Autodesk Inventor part; units mm, degrees
ref_plane "YZ Plane" through (0, 0, 0) normal (1, 0, 0) x (0, 1, 0)
ref_plane "XZ Plane" through (0, 0, 0) normal (0, 1, 0) x (-1, 0, 0)
ref_plane "XY Plane" through (0, 0, 0) normal (0, 0, 1) x (1, 0, 0)
sketch "Sketch1" plane through (0, 0, 0) normal (0, 0, 1) x (1, 0, 0)
  line L0 (0, 0) -> (25.4, 0)
  line L1 (25.4, 0) -> (25.4, 6.35)
  line L2 (25.4, 6.35) -> (0, 6.35)
  line L3 (0, 6.35) -> (0, 0)
  dimension "d0" = 25.4
  dimension "d1" = 6.35
extrude "Extrusion1" add sketch "Sketch1" along normal blind 25.4
sketch "Sketch2" plane through (0, 6.35, 0) normal (0, 1, 0) x (1, 0, 0)
  line L0 (0, 0) -> (25.4, 0)
  line L1 (12.7, 0) -> (12.7, -25.4)
  line L2 (0, -25.4) -> (25.4, -25.4)
  line L3 (0, 0) -> (0, -25.4)
  line L4 (0, -12.7) -> (25.4, -12.7)
  line L5 (25.4, 0) -> (25.4, -25.4)
  line L6 (12.7, -12.7) -> (12.7, -6.35)
  line L7 (12.7, -12.7) -> (12.7, -19.05)
  circle A0 centre (12.7, -6.35) radius 1.5875
  circle A1 centre (12.7, -19.05) radius 1.5875
  dimension "d4" = 6.35
  dimension "d5" = 6.35
  dimension "d6" = 3.175
  dimension "d7" = 3.175
extrude "Extrusion2" cut sketch "Sketch2" against normal blind 25.4 contours A0 L1 | L1 A0 | A1 L1 | L1 A1
sketch "Sketch3" plane through (25.4, 0, 0) normal (1, 0, 0) x (0, 0, -1)
  line L0 (-25.4, 0) -> (-25.4, 6.35)
  line L1 (-25.4, 3.175) -> (0, 3.175)
  line L2 (0, 0) -> (0, 6.35)
  line L3 (-20.6375, 6.35) -> (-20.6375, 0)
  line L4 (-20.6375, 6.35) -> (-20.6375, 3.175)
  line L5 (-4.7625, 6.35) -> (-4.7625, 0)
  line L6 (-4.7625, 6.35) -> (-4.7625, 3.175)
hole "Hole1" at (25.4, 3.175, 20.6375) at (25.4, 3.175, 4.7625) direction (-1, 0, 0) diameter 2.6416 depth 8.255 tip angle 118
properties part number "ElectronicsPlateConnector"
Geometry check sheet. Reference: the model listing, model coordinates, mm. A direction names the side the tool comes from. Coordinates: 2 decimals unless noted, no trailing zeros. Loops run counter-clockwise (first coordinate to the right, second up) from the corner with the lowest first, then second, coordinate; pieces in that order, holes last.
Item 1: Thickness scan on line 1 (Z direction, x = 12.7, y = 2.25); line 2 (X direction, y = 3.25, z = 19.05); line 3 (Z direction, x = 13.25, y = 2). Record the ranges inside material, lowest first.
Item 2: Access from +Z, -Z, +X, -X, +Y, -Y to the whole of each face (thin tool, end or side, straight path). Record for faces 4 (the face through (21.215, 3.117, 6.082)), 5 (the face through (13, 0, 13)).
Item 3: Sectioned sample at A-A, the plane y = 5.25. Count the separate pieces of the cut face and the enclosed holes in it, then the cut area to 3 significant figures.
Item 4: Release check for a two-part mould opening along Z. For faces 1 (the face through (25.4, 3, 13)), 2 (the face through (13, 3, 25.4)), 3 (the face through (13.55, 3.22, 17.71)) record: released by +Z, released by -Z, zero draft, split by the parting line, or undercut.
Item 5: Go/stop test with a flat-tipped pin: pin 1 Ø2 at (y, z) = (3.18, 4.76) entering from +X. Record where the tip stops, or that it passes through.
Item 6: Sectioned sample at B-B, the plane x = 12.7. Record the boundary of the cut face in (y, z), then the cut area to 3 significant figures.
Check result:
1. line 1: z = 0 to 4.76, 7.94 to 17.46, 20.64 to 25.4
1. line 2: x = 0 to 11.11, 14.29 to 25.4
1. line 3: z = 0 to 4.86, 7.84 to 17.56, 20.54 to 25.4
2. face 4: +X
2. face 5: +Z, -Z, +X, -X, -Y
3. separate pieces: 1
3. enclosed holes: 2
3. area: 629 mm2
4. face 1: zero draft
4. face 2: released by +Z
4. face 3: undercut
5. pin 1: stops at x = 16.96
6. outline: (0, 0) - (6.35, 0) - (6.35, 4.76) - (0, 4.76) - close; (0, 7.94) - (6.35, 7.94) - (6.35, 17.46) - (0, 17.46) - close; (0, 20.64) - (6.35, 20.64) - (6.35, 25.4) - (0, 25.4) - close
6. area: 121 mm2
